The listing builds one solid part. Answer for the finished solid, in the listing's coordinates (mm). A direction names the side the tool comes from. Round coordinates to 2 decimals unless told otherwise and drop trailing zeros. Write each loop counter-clockwise with the first axis right and the second up, starting at its lowest first coordinate (ties: lowest second). Pieces come first, ordered by that corner, then holes.
Item 1: Find section C-C on z = 5.5. Give the number of separate pieces and of enclosed holes in the cut face, then the cut area to 3 significant figures.
Item 2: Find the intervals of material crossed by probe 1 along Y at (x, z) = (176, 5.25); probe 2 along Y at (x, z) = (343, 8.75); probe 3 along X at (y, z) = (109.5, 8.5), in increasing order.
Item 3: Find section A-A on y = 243.5. Give the vertices of the cut face in (x, z).
Item 4: A tool of negligible diameter and unlimited length cuts with its end or side. For faces 1 (the face through (325, 332.141, 5)), 2 (the face through (169.187, 239, 5)), 3 (the face through (144.621, 105, 5)), from which of +Z, -Z, +X, -X, +Y, -Y can it reach the whole face along a straight path? Write none if from no direction.
Item 5: Each of these flat-tipped pins is pushed along its axis until it touches: pin 1 (24 mm diameter, centred on x = 52.64, y = 2.65, fed in from +Z); pin 2 (3 mm diameter, centred on x = -39.5, z = 3.5, fed in from +Y); pin 3 (5 mm diameter, centred on x = 115.5, z = 6.5, fed in from +Y); pin 4 (3 mm diameter, centred on y = 225.5, z = 4, fed in from -X). Where does it stop, or does it pass through?
Item 6: Find section D-D on x = -3. Give the vertices of the cut face in (y, z).
Item 7: Find section B-B on x = 102.5. Give the vertices of the cut face in (y, z), then the cut area to 3 significant figures.
Item 8: For a pull along Y with two mould halves and no side action, classify faces 4 (the face through (371.945, 185, 5)), 5 (the face through (349.7, 70.67, 4.93)), 6 (the face through (-22, 55.17, 5)) as +Y half, -Y half, draft (parallel to the pull), parting line (faces both ways), or undercut.
```python
from build123d import *

# Parameters (mm, degrees)
SKETCH1_R           = 7.5
SKETCH1_R_2         = 10
BOSS_EXTRUDE1_DEPTH = 10


with BuildPart() as part:
    # Sketch1 → Boss-Extrude1 (new body)
    with BuildSketch(Plane.XY):
        Polygon((-98.05511991, -17.859318996), (322.382476836, -17.859318996), (322.382476836, 42.140681004), (371.94488009, 42.140681004), (371.94488009, 332.140681004), (277.025034275, 332.140681004), (169.187054595, 271.975052979), (169.187054595, 205.170044114), (30.5872252, 55.170044114), (-76.268588622, 55.170044114), (-98.05511991, 43.014768752), align=None)
        with Locations((-15.752224544, 2.649813362)):
            Circle(SKETCH1_R, mode=Mode.SUBTRACT)
        with Locations((-75.556801399, 2.649813362)):
            Circle(SKETCH1_R, mode=Mode.SUBTRACT)
        with Locations((52.636779721, 2.649813362)):
            Circle(SKETCH1_R, mode=Mode.SUBTRACT)
        with Locations((132.925934878, 2.649813362)):
            Circle(SKETCH1_R, mode=Mode.SUBTRACT)
        with Locations((169.187054595, 83.663978495)):
            Circle(SKETCH1_R, mode=Mode.SUBTRACT)
        with Locations((169.187054595, 125.357526882)):
            Circle(SKETCH1_R, mode=Mode.SUBTRACT)
        with Locations((169.187054595, 175.474014337)):
            Circle(SKETCH1_R, mode=Mode.SUBTRACT)
        with Locations((229.870255563, 265.671146953)):
            Circle(SKETCH1_R_2, mode=Mode.SUBTRACT)
        with Locations((229.870255563, 102.825256229)):
            Circle(SKETCH1_R_2, mode=Mode.SUBTRACT)
        with Locations((340.159565259, 299.323240315)):
            Circle(SKETCH1_R_2, mode=Mode.SUBTRACT)
        with Locations((340.159565259, 67.667528684)):
            Circle(SKETCH1_R_2, mode=Mode.SUBTRACT)
        with BuildLine():
            Line((312.226028305, 265.671146953), (312.226028305, 115.671146953))
            ThreePointArc((312.226028305, 115.671146953), (288.591642629, 92.036761277), (264.957256952, 115.671146953))
            Line((264.957256952, 115.671146953), (264.957256952, 265.671146953))
            ThreePointArc((264.957256952, 265.671146953), (288.591642629, 289.30553263), (312.226028305, 265.671146953))
        make_face(mode=Mode.SUBTRACT)
        Polygon((78.874891909, 71.306483913), (144.620819019, 137.052411023), (144.620819019, 71.306483913), align=None, mode=Mode.SUBTRACT)
    extrude(amount=BOSS_EXTRUDE1_DEPTH)


solid = part.part
```
Check values:
1. separate pieces: 1
1. enclosed holes: 13
1. area: 81,000 mm2
2. probe 1: y = -17.86 to 80.53, 86.8 to 122.22, 128.49 to 172.34, 178.61 to 275.78
2. probe 2: y = 42.14 to 58.08, 77.26 to 289.74, 308.91 to 332.14
2. probe 3: x = 80.79 to 117.07, 144.62 to 222.42, 237.32 to 265.78, 311.41 to 371.94
3. outline: (169.19, 0) - (264.96, 0) - (264.96, 10) - (169.19, 10) - close; (312.23, 0) - (371.94, 0) - (371.94, 10) - (312.23, 10) - close
4. face 1: +Z, -Z, +X, -X, +Y
4. face 2: +Z, -Z, -X, +Y
4. face 3: +Z, -Z
5. pin 1: stops at z = 10
5. pin 2: stops at y = 55.17
5. pin 3: stops at y = 149.77
5. pin 4: stops at x = 169.19
6. outline: (-17.86, 0) - (55.17, 0) - (55.17, 10) - (-17.86, 10) - close
7. outline: (-17.86, 0) - (71.31, 0) - (71.31, 10) - (-17.86, 10) - close; (94.93, 0) - (133, 0) - (133, 10) - (94.93, 10) - close
7. area: 1,270 mm2
8. face 4: draft
8. face 5: undercut
8. face 6: +Y half
